Read the model definition and answer for the solid it produces. Units are mm, in the model's axes. Face numbers are marked on the shaded views. A direction names the side the tool comes from. Round coordinates to 2 decimals unless told otherwise and drop trailing zeros. Order: outer loops, then holes, each group sorted by start corner. A loop starts at its lowest first (then second) coordinate and runs counter-clockwise, first axis right, second up. Notation, with made-up numbers: (70.5, 16.5) - (128.5, 16.5) arc R20 cw to (128.5, 34.5) - close; hole circle Ø3 at (81, -21). An arc over 180 degrees is marked (long way). One line per question, with ' | ' between items. Start each with the question number.
1) The part is cut by section B-B, the plane y = 44.5. Give the vertices of the cut face in (x, z).
2) Flat-ended cylindrical pins translate along their axes: pin 1 (6 mm diameter, centred on y = 24, z = -22, fed in from -X); pin 2 (6 mm diameter, centred on y = 5, z = 34.5, fed in from +X); pin 3 (4 mm diameter, centred on x = 21.5, y = 15, fed in from +Z). Find the tip coordinate at first contact, or state that the pin passes through.
3) For the marked faces 1, 2 and 3, determine the directions among +Z, -Z, +X, -X, +Y, -Y from which every point of the face is accessible in a straight line to the end or side of a thin tool.
4) The part is cut by section A-A, the plane z = 0. Give the vertices of the cut face in (x, y), plus the area to 3 significant figures.
5) Straight lines are drawn through the part: line 1 (X direction, y = 34, z = 0); line 2 (X direction, y = 24.5, z = 0); line 3 (Z direction, x = 0, y = -2.5). For each, find the intervals that lie inside material, in ascending order. Write a range as from..to.
6) The part is cut by section C-C, the plane z = 23.5. Give the vertices of the cut face in (x, y).
7) The part is cut by section D-D, the plane y = 0. Give the vertices of the cut face in (x, z), plus the area to 3 significant figures.
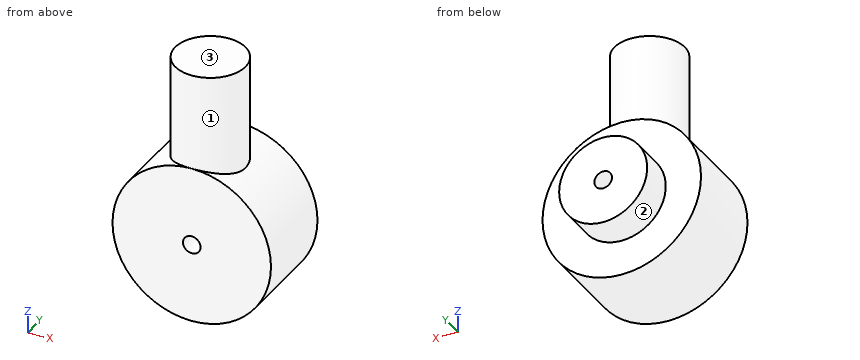
Autodesk Inventor part; units mm, degrees
ref_plane "YZ Plane" through (0, 0, 0) normal (1, 0, 0) x (0, 1, 0)
ref_plane "XZ Plane" through (0, 0, 0) normal (0, 1, 0) x (-1, 0, 0)
ref_plane "XY Plane" through (0, 0, 0) normal (0, 0, 1) x (1, 0, 0)
sketch "Sketch1" plane through (0, 0, 0) normal (0, 0, 1) x (1, 0, 0)
  circle A0 centre (0, 0) radius 20
  dimension "d0" = 40
extrude "Extrusion1" add sketch "Sketch1" along normal blind 100
sketch "Sketch2" plane through (0, 0, 0) normal (0, 1, 0) x (-1, 0, 0)
  line L0 (20, 0) -> (-20, 0)
  circle A0 centre (0, 0) radius 45
  dimension "d3" = 90
extrude "Extrusion2" add sketch "Sketch2" along normal blind 30 and the other way blind 20
sketch "Sketch4" plane through (0, 30, 0) normal (0, 1, 0) x (1, 0, 0)
  circle A0 centre (0, 0) radius 5
  dimension "d9" = 10
extrude "Extrusion4" cut sketch "Sketch4" along normal through all both and the other way through all
sketch "Sketch6" plane through (0, 30, 0) normal (0, 1, 0) x (1, 0, 0)
  circle A0 centre (0, 0) radius 5
  circle A1 centre (0, 0) radius 25
  circle A2 centre (0, 0) radius 15
  dimension "d15" = 50
  dimension "d16" = 30
extrude "Extrusion6" add sketch "Sketch6" along normal blind 20 contours A1 | A2
properties part number "End Link 2"
Values:
1) outline: circle Ø50 at (0, 0); hole circle Ø10 at (0, 0)
2) pin 1: stops at x = -40.79 | pin 2: stops at x = 32.14 | pin 3: stops at z = 40.56
3) face 1: +Z | face 2: +Y | face 3: +Z, +X, -X, +Y, -Y
4) outline: (-45, -20) - (-5, -20) - (-5, 50) - (-25, 50) - (-25, 30) - (-45, 30) - close; (5, -20) - (45, -20) - (45, 30) - (25, 30) - (25, 50) - (5, 50) - close | area: 4,800 mm^2
5) line 1: x = -25..-5, 5..25 | line 2: x = -45..-5, 5..45 | line 3: z = -45..-5, 5..100
6) outline: (-38.38, -20) - (38.38, -20) - (38.38, 30) - (8.53, 30) - (8.53, 50) - (-8.53, 50) - (-8.53, 30) - (-38.38, 30) - close
7) outline: (-20, 40.31) arc R45 ccw (long way) to (20, 40.31) - (20, 100) - (-20, 100) - close; hole circle Ø10 at (0, 0) | area: 8,540 mm^2
